Source: CAD feature listing. Evaluate the final solid. Frame: model axes, mm. A direction names the side the tool comes from. Round coordinates to 2 decimals unless told otherwise and drop trailing zeros. Order: outer loops, then holes, each group sorted by start corner. A loop starts at its lowest first (then second) coordinate and runs counter-clockwise, first axis right, second up. Notation, with made-up numbers: (55, 85.5) - (92, 85.5) arc R24 ccw to (92, 123.5) - close; hole circle Ø11 at (57, -26.5). An arc over 180 degrees is marked (long way). Use one line per item in the form item = value. Start each with the question number.
Q1. Ray query, line 1 (Y direction, x = -21.5, z = 9.75); line 2 (Y direction, x = -43, z = 11.25); line 3 (X direction, y = -11.5, z = 6). Return the intervals inside material, ascending. Write a range as [from, to].
Q2. Cut plane B-B, the plane z = 11.5. Give the number of separate pieces and of enclosed holes in the cut face, and give its area (3 significant figures).
Q3. Draft query along X for faces 1 (the cylindrical face through (-36.975, 11.422, 1.016)), 2 (the flat face through (-37, 2, 0)), 3 (the flat face through (1, 1, 9)). Return one class per face: released by +X, released by -X, zero draft, split by the parting line, or undercut.
Q4. Pin query (flat end, axial travel): pin 1 Ø0.8 at (x, y) = (-75.5, 9) entering from +Z; pin 2 Ø3 at (x, z) = (-23.5, 14) entering from +Y; pin 3 Ø6 at (x, y) = (-55.5, -11) entering from +Z. Return the tip coordinate at first contact, or that it passes through.
Q5. Cut plane C-C, the plane y = 7. Return the cut outline in (x, z).
Q6. Set-up query: faces 4 (the flat face through (-76, 2, 9)), 5 (the flat face through (-75, -3, 10)). Return all of +Z, -Z, +X, -X, +Y, -Y with unobstructed straight access to the full face (end or side cutting, diameter ignored); none if empty.
from build123d import *

# Parameters (mm, degrees)
F0_W     = 40
F0_H     = 18.241094
F1_DEPTH = 1
F3_DEPTH = 75
F5_DEPTH = 1


with BuildPart() as f1:
    # F0 (on Right) → F1 (new body)
    with BuildSketch(Plane.YZ):
        with Locations((1.416398, 9.120547)):
            Rectangle(F0_W, F0_H)
    extrude(amount=F1_DEPTH)

    # F2 (on Right) → F3 (join)
    with BuildSketch(Plane.YZ):
        with BuildLine():
            Line((-18.647401, 0), (21.388335, 0))
            Line((21.388335, 0), (21.388335, 16.275622))
            Line((21.388335, 16.275622), (20.506265, 16.275622))
            Line((20.506265, 16.275622), (20.506265, 10.329797))
            ThreePointArc((20.506265, 10.329797), (11.217281, 1.01272), (1.872196, 10.273525))
            Line((1.872196, 10.273525), (1.850361, 13.888834))
            Line((1.850361, 13.888834), (0.837944, 13.88272))
            Line((0.837944, 13.88272), (0.859742, 10.273525))
            ThreePointArc((0.859742, 10.273525), (-8.638272, 0.863686), (-17.842658, 10.560934))
            Line((-17.842658, 10.560934), (-17.842658, 16.275622))
            Line((-17.842658, 16.275622), (-18.647401, 16.275622))
            Line((-18.647401, 16.275622), (-18.647401, 0))
        make_face()
    extrude(amount=-F3_DEPTH)

    # F4 (on face) → F5 (join)
    with BuildSketch(Plane(origin=(-75, 0, 0), x_dir=(0, -1, 0), z_dir=(-1, 0, 0))):
        with BuildLine():
            Line((18.586515, 0), (18.586515, 16.275622))
            Line((18.586515, 16.275622), (17.842658, 16.275622))
            Line((17.842658, 16.275622), (17.842658, 10.560934))
            ThreePointArc((17.842658, 10.560934), (8.638272, 0.863686), (-0.859742, 10.273525))
            Line((-0.859742, 10.273525), (-0.837944, 13.88272))
            Line((-0.837944, 13.88272), (-1.850361, 13.888834))
            Line((-1.850361, 13.888834), (-1.872196, 10.273525))
            ThreePointArc((-1.872196, 10.273525), (-11.217281, 1.01272), (-20.506265, 10.329797))
            Line((-20.506265, 10.329797), (-20.506265, 16.275622))
            Line((-20.506265, 16.275622), (-21.388335, 16.275622))
            Line((-21.388335, 16.275622), (-21.388335, 0))
            Line((-21.388335, 0), (18.586515, 0))
        make_face()
        with BuildLine():
            Line((18.586515, 16.275622), (18.586515, 18.236505))
            Line((18.586515, 18.236505), (-21.388335, 18.236505))
            Line((-21.388335, 18.236505), (-21.388335, 16.275622))
            Line((-21.388335, 16.275622), (-20.506265, 16.275622))
            Line((-20.506265, 16.275622), (-20.506265, 10.329797))
            ThreePointArc((-20.506265, 10.329797), (-11.217281, 1.01272), (-1.872196, 10.273525))
            Line((-1.872196, 10.273525), (-1.850361, 13.888834))
            Line((-1.850361, 13.888834), (-0.837944, 13.88272))
            Line((-0.837944, 13.88272), (-0.859742, 10.273525))
            ThreePointArc((-0.859742, 10.273525), (8.638272, 0.863686), (17.842658, 10.560934))
            Line((17.842658, 10.560934), (17.842658, 16.275622))
            Line((17.842658, 16.275622), (18.586515, 16.275622))
        make_face()
    extrude(amount=F5_DEPTH)


solid = f1.part
Completed:
q1.line_1 = [-18.65, -17.84], [0.85, 1.89], [20.49, 21.39]
q1.line_2 = [-18.65, -17.84], [0.85, 1.87], [20.51, 21.39]
q1.line_3 = [-76, -75], [0, 1]
q2.separate_pieces = 1
q2.enclosed_holes = 2
q2.area = 282 mm2
q3.face_1 = undercut
q3.face_2 = zero draft
q3.face_3 = released by +X
q4.pin_1 = 18.24
q4.pin_2 = 21.39
q4.pin_3 = 2.65
q5.outline = (-76, 0) - (1, 0) - (1, 18.24) - (0, 18.24) - (0, 2.01) - (-75, 2.01) - (-75, 18.24) - (-76, 18.24) - close
q6.face_4 = +Z, -Z, -X, +Y, -Y
q6.face_5 = +Z
